The model under review builds one solid part; all positions refer to its coordinate system, in mm. Face numbers are marked on the shaded views. A direction names the side the tool comes from. Give positions to 0.01 mm unless a question says otherwise; leave off trailing zeros. Order: outer loops, then holes, each group sorted by start corner. A loop starts at its lowest first (then second) coordinate and runs counter-clockwise, first axis right, second up.
Autodesk Inventor part; units mm, degrees
ref_plane "YZ Plane" through (0, 0, 0) normal (1, 0, 0) x (0, 1, 0)
ref_plane "XZ Plane" through (0, 0, 0) normal (0, 1, 0) x (-1, 0, 0)
ref_plane "XY Plane" through (0, 0, 0) normal (0, 0, 1) x (1, 0, 0)
sketch "Base" plane through (0, 0, 0) normal (0, 0, 1) x (1, 0, 0)
  spline S0 degree 3 poles (29.6992, 1.1773) (29.7109, 1.3423) (29.6903, 1.508) (29.5867, 1.8221) (29.5048, 1.9675) (29.2897, 2.2188) (29.1586, 2.3222) (28.9221, 2.4433) (28.8277, 2.4783) (28.6327, 2.5254) (28.5327, 2.5373) (28.4324, 2.5373) knots 0 0 0 0 0.049612 0.049612 0.099224 0.099224 0.148836 0.148836 0.178932 0.178932 0.209028 0.209028 0.209028 0.209028
  line L0 (1.5557, 2.5369) -> (28.4324, 2.5373)
  spline S1 degree 3 poles (1.5557, 2.5369) (1.3904, 2.5369) (1.2266, 2.5046) (0.9206, 2.379) (0.7813, 2.287) (0.5459, 2.0546) (0.452, 1.9166) (0.3443, 1.6634) (0.3145, 1.5572) (0.2831, 1.3399) (0.2816, 1.2297) (0.2942, 1.1206) knots 0 0 0 0 0.049612 0.049612 0.099224 0.099224 0.148836 0.148836 0.181775 0.181775 0.214715 0.214715 0.214715 0.214715
  arc A0 (0, 0) -> (0.2942, 1.1206) centre (-1.2879, 0.9371) ccw
  line L1 (30.1691, 0) -> (0, 0)
  arc A1 (29.6992, 1.1773) -> (30.1691, 0) centre (31.151, 1.0743) ccw
  spline S2 degree 3 poles (-2.6437, -23.0226) (-2.6437, -23.1879) (-2.6114, -23.3517) (-2.4858, -23.6576) (-2.3938, -23.7968) (-2.1615, -24.0323) (-2.0234, -24.1261) (-1.7866, -24.227) (-1.6982, -24.2538) (-1.5172, -24.2877) (-1.4252, -24.2948) (-1.3332, -24.2919) knots 0 0 0 0 0.049602 0.049602 0.099207 0.099207 0.148822 0.148822 0.176438 0.176438 0.204053 0.204053 0.204053 0.204053
  arc A2 (0, -24.9362) -> (-1.3332, -24.2919) centre (-1.2826, -25.8888) ccw
  line L2 (0, 0) -> (0, -24.9362)
  arc A3 (-1.3355, -0.6549) -> (0, 0) centre (-1.2879, 0.9371) ccw
  spline S3 degree 3 poles (-1.3355, -0.6549) (-1.5008, -0.65) (-1.6656, -0.6774) (-1.9753, -0.7938) (-2.1173, -0.8817) (-2.3596, -1.107) (-2.4576, -1.2422) (-2.5652, -1.4755) (-2.5945, -1.5626) (-2.6338, -1.7415) (-2.6437, -1.8328) (-2.6437, -1.9244) knots 0 0 0 0 0.049634 0.049634 0.099263 0.099263 0.148881 0.148881 0.176354 0.176354 0.203827 0.203827 0.203827 0.203827
  line L3 (-2.6437, -23.0226) -> (-2.6437, -1.9244)
  spline S4 degree 3 poles (28.1591, -27.4789) (28.3245, -27.4789) (28.4883, -27.4466) (28.7943, -27.3211) (28.9335, -27.229) (29.1689, -26.9966) (29.2628, -26.8586) (29.3703, -26.6061) (29.3999, -26.5007) (29.4315, -26.285) (29.4334, -26.1755) (29.4212, -26.0671) knots 0 0 0 0 0.049612 0.049612 0.099224 0.099224 0.148836 0.148836 0.181546 0.181546 0.214256 0.214256 0.214256 0.214256
  arc A4 (31.1912, -24.3016) -> (29.4212, -26.0671) centre (31.0088, -25.8888) ccw
  spline S5 degree 3 poles (31.1912, -24.3016) (31.3556, -24.3204) (31.5221, -24.307) (31.8405, -24.2172) (31.9894, -24.1416) (32.2499, -23.9376) (32.3589, -23.8111) (32.4948, -23.5721) (32.5363, -23.4703) (32.5923, -23.2585) (32.6065, -23.1495) (32.6065, -23.0399) knots 0 0 0 0 0.049634 0.049634 0.099263 0.099263 0.148881 0.148881 0.18174 0.18174 0.214599 0.214599 0.214599 0.214599
  line L4 (32.6065, -1.6448) -> (32.6065, -23.0399)
  spline S6 degree 3 poles (32.6065, -1.6448) (32.6065, -1.4795) (32.5742, -1.3157) (32.4486, -1.0098) (32.3566, -0.8705) (32.1243, -0.6351) (31.9862, -0.5412) (31.7423, -0.4373) (31.6462, -0.4092) (31.4495, -0.376) (31.3495, -0.371) (31.2499, -0.3778) knots 0 0 0 0 0.049602 0.049602 0.099206 0.099206 0.14882 0.14882 0.178752 0.178752 0.208681 0.208681 0.208681 0.208681
  arc A5 (30.1691, 0) -> (31.2499, -0.3778) centre (31.151, 1.0743) ccw
  line L5 (30.1691, -22.3113) -> (30.1691, 0)
  line L6 (27.5442, -22.3113) -> (30.1691, -22.3113)
  line L7 (27.5442, -24.9362) -> (27.5442, -22.3113)
  line L8 (0, -24.9362) -> (27.5442, -24.9362)
  arc A6 (0.305, -26.0673) -> (0, -24.9362) centre (-1.2826, -25.8888) ccw
  spline S7 degree 3 poles (0.305, -26.0673) (0.2866, -26.2317) (0.3003, -26.398) (0.3909, -26.7161) (0.4669, -26.8648) (0.6714, -27.1247) (0.7981, -27.2334) (1.037, -27.3685) (1.1385, -27.4097) (1.3494, -27.4652) (1.458, -27.4793) (1.5671, -27.4793) knots 0 0 0 0 0.049612 0.049612 0.099224 0.099224 0.148836 0.148836 0.181555 0.181555 0.214273 0.214273 0.214273 0.214273
  line L9 (28.1591, -27.4789) -> (1.5671, -27.4793)
  point P0 (30.1691, 0)
  point P1 (30.1691, 0)
extrude "BaseFeature" add sketch "Base" along normal blind 3.81
extrude "LogoFeature" add sketch "Base" against normal blind 5.08 contours L5 L6 L7 L8 L2 L1
sketch "LogoDetail" plane through (0, 0, -5.08) normal (0, 0, -1) x (-1, 0, 0)
  line L0 (-18.374, -7.8746) -> (-22.2945, -7.8746)
  line L1 (-27.5442, -22.3113) -> (-13.1243, -22.3113)
  line L2 (-22.2945, -17.0616) -> (-18.374, -17.0616)
  line L3 (-13.1243, -2.6249) -> (-27.5442, -2.6249)
  line L4 (-22.2945, -7.8746) -> (-22.2945, -17.0616)
  line L5 (-18.374, -17.0616) -> (-18.374, -7.8746)
  line L6 (-30.1691, -22.3113) -> (-30.1691, 0)
  line L7 (-27.5442, -2.6249) -> (-27.5442, -22.3113)
  line L8 (-13.1243, -22.3113) -> (-13.1243, -2.6249)
  line L9 (-30.1691, 0) -> (0, 0)
  line L10 (0, -24.9362) -> (-27.5442, -24.9362)
  line L11 (-7.8746, -2.6249) -> (-7.8746, -22.3113)
  line L12 (-2.6249, -22.3113) -> (-2.6249, -2.6249)
  line L13 (-7.8746, -22.3113) -> (-2.6249, -22.3113)
  line L14 (-2.6249, -2.6249) -> (-7.8746, -2.6249)
  line L15 (-27.5442, -24.9362) -> (-27.5442, -22.3113)
  line L16 (-27.5442, -22.3113) -> (-30.1691, -22.3113)
  line L17 (0, 0) -> (0, -24.9362)
  line L18 (-30.1691, -22.3113) -> (-30.1691, -24.9362)
  line L19 (-30.1691, -24.9362) -> (-27.5442, -24.9362)
  line L20 (0, 0) -> (-30.1691, 0)
  line L21 (-30.1691, 0) -> (-30.1691, -22.3113)
  dimension "d4" = 3.9205
  dimension "d5" = 5.2497
  dimension "d6" = 5.2497
  dimension "d7" = 5.2497
  dimension "d8" = 2.6249
  dimension "d9" = 5.2497
  dimension "d10" = 5.2497
  dimension "d11" = 2.6249
  dimension "d12" = 2.6249
  dimension "d13" = 2.6249
  dimension "d14" = 24.9362
  dimension "d15" = 27.5443
  dimension "d16" = 5.2497
extrude "LogoDetailFeature" cut sketch "LogoDetail" against normal blind 5.08 contours L5 L2 L4 L0 | L16 L6 L9 L17 L10 L15
properties part number "switchback-logo"
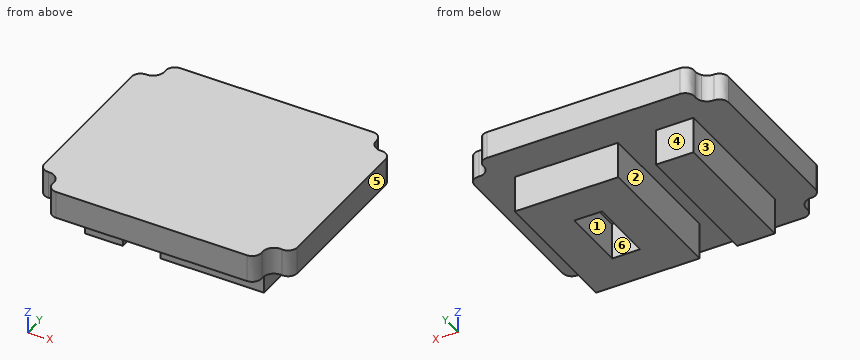
Item 1: For line 1 (X direction, y = -16, z = -3.5); line 2 (X direction, y = -21.5, z = -1); line 3 (Z direction, x = 17, y = -1), list the stretches that pass through material, from the lowest coordinate up.
Values found:
line 1: x = 2.62 to 7.87, 13.12 to 18.37, 22.29 to 27.54
line 2: x = 2.62 to 7.87, 13.12 to 27.54
line 3: z = 0 to 3.81
Item 2: Take a section at D-D (y = -19). Give the boundary of the cut face in (x, z), and give its area (3 significant figures).
Values found:
outline: (-2.64, 0) - (2.62, 0) - (2.62, -5.08) - (7.87, -5.08) - (7.87, 0) - (13.12, 0) - (13.12, -5.08) - (27.54, -5.08) - (27.54, 0) - (32.61, 0) - (32.61, 3.81) - (-2.64, 3.81) - close
area: 234 mm2
Item 3: For the marked faces 1, 2 and 3, list the 3-axis set-ups (+Z, -Z, +X, -X, +Y, -Y) from which the entire face can be reached by the end or side of a thin tool; tool diameter is ignored.
Values found:
face 1: -Z
face 2: -Z, +Y, -Y
face 3: -Z, -X, +Y, -Y
Item 4: Take a section at A-A (z = -2). Give the boundary of the cut face in (x, y).
Values found:
outline: (2.62, -22.31) - (7.87, -22.31) - (7.87, -2.62) - (2.62, -2.62) - close; (13.12, -22.31) - (27.54, -22.31) - (27.54, -2.62) - (13.12, -2.62) - close; hole (18.37, -17.06) - (22.29, -17.06) - (22.29, -7.87) - (18.37, -7.87) - close
Item 5: Take a section at B-B (y = -14). Give the boundary of the cut face in (x, z), and give its area (3 significant figures).
Values found:
outline: (-2.64, 0) - (2.62, 0) - (2.62, -5.08) - (7.87, -5.08) - (7.87, 0) - (13.12, 0) - (13.12, -5.08) - (18.37, -5.08) - (18.37, 0) - (22.29, 0) - (22.29, -5.08) - (27.54, -5.08) - (27.54, 0) - (32.61, 0) - (32.61, 3.81) - (-2.64, 3.81) - close
area: 214 mm2
Item 6: Draft analysis for pull direction Y (two halves, no side actions). For the marked faces 4, 5 and 6, state which applies: released by +Y, released by -Y, zero draft, split by the parting line, or undercut.
Values found:
face 4: released by +Y
face 5: zero draft
face 6: undercut
Item 7: Clearance check with flat-ended pins moving along their axes: pin 1 Ø1.5 at (y, z) = (-9.5, -2) entering from +X; pin 2 Ø3 at (x, z) = (21, -2) entering from -Y; pin 3 Ø5 at (x, z) = (20.5, -4) entering from +Y. State where each tip first meets the part, or that it passes through.
Values found:
pin 1: stops at x = 27.54
pin 2: stops at y = -22.31
pin 3: stops at y = -2.62
Item 8: Take a section at C-C (x = 23). Give the boundary of the cut face in (y, z).
Values found:
outline: (-27.48, 0) - (-22.31, 0) - (-22.31, -5.08) - (-2.62, -5.08) - (-2.62, 0) - (2.54, 0) - (2.54, 3.81) - (-27.48, 3.81) - close
